For this review, take the finished solid that the model builds, in its own axes (mm). A direction names the side the tool comes from. Give positions to 0.01 mm unless a question says otherwise; leave off trailing zeros. Loops run counter-clockwise (first coordinate to the right, second up) from the corner with the lowest first, then second, coordinate; pieces in that order, holes last. Notation, with made-up numbers: (53, 82) - (96, 82) arc R21 cw to (96, 91) - close; hole circle Ø5 at (79.25, 14). An arc over 180 degrees is marked (long way). Answer in a Markdown table with one row per item.
```python
from build123d import *

# Parameters (mm, degrees)
SKETCH4_R                  = 22.225
BOSS_EXTRUDE1_DEPTH        = 30.48
F_7_8_14_UNF_FITTING_D     = 20.6375
F_7_8_14_UNF_FITTING_DEPTH = 49.784
F_7_8_14_UNF_FITTING_TIP   = 6.200130513


with BuildPart() as part:
    # Sketch1 → Revolve1 (revolve)
    with BuildSketch(Plane(origin=(0, 0, 0), x_dir=(1, 0, 0), z_dir=(0, 1, 0)), mode=Mode.PRIVATE) as revolve1_sk:
        with BuildLine():
            Line((0, 0), (31.75, 0))
            Line((31.75, 0), (31.75, 6.35))
            Line((31.75, 6.35), (38.1, 6.35))
            ThreePointArc((38.1, 6.35), (65.074334034, 33.724356705), (74.93, 70.870499843))
            Line((74.93, 70.870499843), (74.93, 704.85))
            ThreePointArc((74.93, 704.85), (52.983511114, 757.833511114), (0, 779.78))
            Line((0, 779.78), (0, 776.605))
            ThreePointArc((0, 776.605), (50.738447084, 755.588447084), (71.755, 704.85))
            Line((71.755, 704.85), (71.755, 70.870499843))
            ThreePointArc((71.755, 70.870499843), (63.375644219, 37.220719089), (40.194614109, 11.43))
            Line((40.194614109, 11.43), (26.67, 11.43))
            Line((26.67, 11.43), (26.67, 5.08))
            Line((26.67, 5.08), (0, 5.08))
            Line((0, 5.08), (0, 0))
        make_face()
    revolve(revolve1_sk.sketch.rotate(Axis((0, 0, -704.85), (0, 0, 1)), 180), axis=Axis((0, 0, -704.85), (0, 0, 1)))

    # Sketch4 → Boss-Extrude1 (add)
    with BuildSketch(Plane.XY):
        with Locations(Location((0, 0, 0), (0, 0, 180))):
            Circle(SKETCH4_R)
    extrude(amount=BOSS_EXTRUDE1_DEPTH)

    # 7/8-14 UNF Fitting
    with Locations(Plane(origin=(-8.590582688, 4.968077157, 30.48), x_dir=(1, 0, 0), z_dir=(0, 0, 1))):
        with Locations((8.590582688, -4.968077157)):
            Hole(F_7_8_14_UNF_FITTING_D / 2, depth=F_7_8_14_UNF_FITTING_DEPTH)
            with Locations((0, 0, -(F_7_8_14_UNF_FITTING_DEPTH + F_7_8_14_UNF_FITTING_TIP / 2))):  # 118° drill point
                Cone(0, F_7_8_14_UNF_FITTING_D / 2, F_7_8_14_UNF_FITTING_TIP, mode=Mode.SUBTRACT)


solid = part.part
```
1. Mouldability with a two-part tool opening along X and no side actions: class faces 1 (the face through (6.883, 30.995, -3.219)), 2 (the face through (-11, 0, -5.08)), 3 (the face through (-5, 10, 30.48)) as released by +X, released by -X, zero draft, split by the parting line, or undercut.
Values:
| item | result |
|---|---|
| face 1 | split by the parting line |
| face 2 | undercut |
| face 3 | zero draft |
2. We need section D-D, the plane z = -54. Give the boundary of the cut face in (x, y).
Values:
| item | result |
|---|---|
| outline | circle Ø146.01 at (0, 0); hole circle Ø139.49 at (0, 0) |
3. Clearance check with flat-ended pins moving along their axes: pin 1 (10 mm diameter, centred on x = 0, z = -426, fed in from +Y); pin 2 (8 mm diameter, centred on x = -36, y = -22, fed in from +Z); pin 3 (3 mm diameter, centred on y = -48.5, z = -546, fed in from -X). State where each tip first meets the part, or that it passes through.
Values:
| item | result |
|---|---|
| pin 1 | stops at y = 74.93 |
| pin 2 | stops at z = -6.4 |
| pin 3 | stops at x = -58.36 |
4. For faces 4 (the face through (16.24, 73.15, -392.3)), 5 (the face through (16.4, -15, 15)), 6 (the face through (3.472, -26.443, -8.211)), list the 3-axis set-ups (+Z, -Z, +X, -X, +Y, -Y) from which the entire face can be reached by the end or side of a thin tool; tool diameter is ignored.
Values:
| item | result |
|---|---|
| face 4 | +Z, -Z |
| face 5 | +Z |
| face 6 | none |
5. We need section C-C, the plane y = -52. Give the boundary of the cut face in (x, z).
Values:
| item | result |
|---|---|
| outline | (-53.95, -704.85) arc R53.95 ccw to (53.95, -704.85) - (53.95, -70.87) arc R53.95 ccw to (-53.95, -70.87) - close; hole (-49.44, -704.85) arc R49.44 ccw to (49.44, -704.85) - (49.44, -70.87) arc R49.44 ccw to (-49.44, -70.87) - close |
6. Wall thickness on line 1 (Y direction, x = 3, z = -623); line 2 (X direction, y = 4, z = -605.5); line 3 (Y direction, x = 0, z = -9): over which ranges is each line inside the solid? List them lowest first. Write a range as [from, to].
Values:
| item | result |
|---|---|
| line 1 | y = [-74.87, -71.69], [71.69, 74.87] |
| line 2 | x = [-74.82, -71.64], [71.64, 74.82] |
| line 3 | y = [-42.27, -26.67], [26.67, 42.27] |
